```python
from build123d import *

# Parameters (mm, degrees)
SKETCH_1_R      = 11
SKETCH_1_R_2    = 1.75
EXTRUDE_1_DEPTH = 3
EXTRUDE_2_DEPTH = 3
EXTRUDE_3_DEPTH = 3
EXTRUDE_4_DEPTH = 3


with BuildPart() as part:
    # 草图1 → 凸台-拉伸1 (new body)
    with BuildSketch(Plane(origin=(0, 0, 0), x_dir=(1, 0, 0), z_dir=(0, 1, 0))):
        Polygon((0, 0), (50, 0), (50, 45), (45, 50), (5, 50), (0, 45), align=None)
        with Locations(Location((25, 25, 0), (0, 0, 270))):
            Circle(SKETCH_1_R, mode=Mode.SUBTRACT)
        with Locations(Location((9.5, 40.5, 0), (0, 0, 270))):
            Circle(SKETCH_1_R_2, mode=Mode.SUBTRACT)
        with Locations(Location((40.5, 40.5, 0), (0, 0, 90))):
            Circle(SKETCH_1_R_2, mode=Mode.SUBTRACT)
        with Locations(Location((40.5, 9.5, 0), (0, 0, 270))):
            Circle(SKETCH_1_R_2, mode=Mode.SUBTRACT)
        with Locations(Location((9.5, 9.5, 0), (0, 0, 90))):
            Circle(SKETCH_1_R_2, mode=Mode.SUBTRACT)
    extrude(amount=EXTRUDE_1_DEPTH)

    # 草图2 → 凸台-拉伸2 (add)
    with BuildSketch(Plane.XY):
        Polygon((0, 0), (50, 0), (50, 48), (45, 53), (5, 53), (0, 48), align=None)
        with BuildLine():
            Line((7.9, 42), (7.9, 12))
            ThreePointArc((7.9, 12), (10, 9.9), (12.1, 12))
            Line((12.1, 12), (12.1, 42))
            ThreePointArc((12.1, 42), (10, 44.1), (7.9, 42))
        make_face(mode=Mode.SUBTRACT)
        with BuildLine():
            Line((37.9, 42), (37.9, 12))
            ThreePointArc((37.9, 12), (40, 9.9), (42.1, 12))
            Line((42.1, 12), (42.1, 42))
            ThreePointArc((42.1, 42), (40, 44.1), (37.9, 42))
        make_face(mode=Mode.SUBTRACT)
    extrude(amount=EXTRUDE_2_DEPTH)

    # 草图3 → 凸台-拉伸3 (add)
    with BuildSketch(Plane.ZY):
        Polygon((0, 3), (-13, 3), (0, 23), align=None)
    extrude(amount=-EXTRUDE_3_DEPTH)

    # 草图4 → 凸台-拉伸4 (add)
    with BuildSketch(Plane(origin=(50, 0, 0), x_dir=(0, 0, -1), z_dir=(1, 0, 0))):
        Polygon((0, 3), (13, 3), (0, 23), align=None)
    extrude(amount=-EXTRUDE_4_DEPTH)


solid = part.part
```
Design review of the part built by this model. Coordinates are the model's own, in mm. A direction names the side the tool comes from. Coordinates: 2 decimals unless noted, no trailing zeros. Order: outer loops, then holes, each group sorted by start corner. A loop starts at its lowest first (then second) coordinate and runs counter-clockwise, first axis right, second up.
1) Clearance check with flat-ended pins moving along their axes: pin 1 (4 mm diameter, centred on y = 17, z = -7, fed in from -X); pin 2 (1.5 mm diameter, centred on y = 30, z = 2, fed in from -X); pin 3 (4.5 mm diameter, centred on x = 40.5, z = -40.5, fed in from +Y); pin 4 (15 mm diameter, centred on x = 27, y = 17.5, fed in from -Z). State where each tip first meets the part, or that it passes through.
2) Wall thickness on line 1 along X through (y, z) = (1.2, -9.5); line 2 along Z through (x, y) = (40, 1); line 3 along Y through (x, z) = (42.5, -28): over which ranges is each line inside the solid? List them lowest first.
3) Take a section at C-C, the plane z = -16.5. Give the boundary of the cut face in (x, y).
4) Take a section at B-B, the plane y = 31.5. Give the boundary of the cut face in (x, z).
5) Take a section at A-A, the plane x = 25. Give the boundary of the cut face in (y, z), and give its area (3 significant figures).
6) For faces 1 (the flat face through (3, 9, -4)), 2 (the flat face through (3, 51, 1)), 3 (the cylindrical face through (10, 44.1, 1.5)), list the 3-axis set-ups (+Z, -Z, +X, -X, +Y, -Y) from which the entire face can be reached by the end or side of a thin tool; tool diameter is ignored.
7) Mouldability with a two-part tool opening along Y and no side actions: class faces 4 (the cylindrical face through (40, 9.9, 1.5)), 5 (the flat face through (25, 1, -50)), 6 (the flat face through (48.52, 12.86, -6.59)) as +Y half, -Y half, draft (parallel to the pull), parting line (faces both ways), or undercut.
8) Take a section at D-D, the plane z = -40.5. Give the boundary of the cut face in (x, y), and give its area (3 significant figures).
Returned:
1. pin 1: passes through
1. pin 2: stops at x = 0
1. pin 3: stops at y = 3
1. pin 4: stops at z = 0
2. line 1: x = 0 to 7.75, 11.25 to 38.75, 42.25 to 50
2. line 2: z = -50 to -42.18, -38.82 to -11.18, -7.82 to 3
2. line 3: y = 0 to 3
3. outline: (0, 0) - (18.02, 0) - (18.02, 3) - (0, 3) - close; (31.98, 0) - (50, 0) - (50, 3) - (31.98, 3) - close
4. outline: (0, 0) - (7.9, 0) - (7.9, 3) - (0, 3) - close; (12.1, 0) - (37.9, 0) - (37.9, 3) - (12.1, 3) - close; (42.1, 0) - (50, 0) - (50, 3) - (42.1, 3) - close
5. outline: (0, -50) - (3, -50) - (3, -36) - (0, -36) - close; (0, -14) - (3, -14) - (3, 0) - (53, 0) - (53, 3) - (0, 3) - close
5. area: 243 mm2
6. face 1: -Z, +Y
6. face 2: +Z, -Z, -X, +Y
6. face 3: +Z, -Z
7. face 4: undercut
7. face 5: draft
7. face 6: +Y half
8. outline: (0, 0) - (7.75, 0) - (7.75, 3) - (0, 3) - close; (11.25, 0) - (38.75, 0) - (38.75, 3) - (11.25, 3) - close; (42.25, 0) - (50, 0) - (50, 3) - (42.25, 3) - close
8. area: 129 mm2
